from build123d import *

# Parameters (mm, degrees)
SKETCH1_R           = 43.2435
BOSS_EXTRUDE1_DEPTH = 1.5875


with BuildPart() as part:
    # Sketch1 → Boss-Extrude1 (new body)
    with BuildSketch(Plane.XY):
        Circle(SKETCH1_R)
        with BuildLine():
            Line((39.84498, 0.79375), (39.84498, -0.79375))
            Line((39.84498, -0.79375), (31.740076574, -0.79375))
            ThreePointArc((31.740076574, -0.79375), (0, -31.75), (-31.740076574, -0.79375))
            Line((-31.740076574, -0.79375), (-39.84498, -0.79375))
            Line((-39.84498, -0.79375), (-39.84498, 0.79375))
            Line((-39.84498, 0.79375), (-31.740076574, 0.79375))
            ThreePointArc((-31.740076574, 0.79375), (0, 31.75), (31.740076574, 0.79375))
            Line((31.740076574, 0.79375), (39.84498, 0.79375))
        make_face(mode=Mode.SUBTRACT)
    extrude(amount=BOSS_EXTRUDE1_DEPTH)


solid = part.part
Input: part model. Units: mm. Frame: model coordinates. A direction names the side the tool comes from. Give positions to 0.01 mm unless a question says otherwise; leave off trailing zeros. Order: outer loops, then holes, each group sorted by start corner. A loop starts at its lowest first (then second) coordinate and runs counter-clockwise, first axis right, second up. Notation, with made-up numbers: (20.5, -11.75) - (64.5, -11.75) arc R15 cw to (64.5, 5.25) - close; hole circle Ø1 at (-7.5, -25). An arc over 180 degrees is marked (long way). Answer as a JSON object with one key per item and string values. Group by question number.
Q1. Cut plane B-B, the plane x = 0. Output: boundary loops of the cut face in (y, z), then the cut area to 3 significant figures.
Q2. Cut plane C-C, the plane y = 5. Output: boundary loops of the cut face in (x, z).
Q3. Line query: probe 1 along Y at (x, z) = (34, 1.25); probe 2 along X at (y, z) = (-14, 0.3); probe 3 along X at (y, z) = (17, 0.7). Output: solid intervals per line, ascending.
Q4. Set-up query: faces 1 (the face through (-0.687, 31.743, 0.783)), 2 (the face through (0, 32, 0)). Return all of +Z, -Z, +X, -X, +Y, -Y with unobstructed straight access to the full face (end or side cutting, diameter ignored); none if empty.
Q5. Mould query, pull axis Y, two halves, no side actions, for faces 3 (the face through (0, 32, 1.588)), 4 (the face through (23.25, 36.46, 0.78)), 5 (the face through (0.687, -31.743, 0.783)). Classes: pulls with the +Y half, pulls with the -Y half, needs draft (parallel to the pull), parting line crosses it, or undercut.
Q6. Cut plane A-A, the plane z = 1.2. Output: boundary loops of the cut face in (x, y), then the cut area to 3 significant figures.
Q7. First-contact query: pin 1 Ø0.8 at (x, z) = (37, 1) entering from +Y. Flat tip, straight axial feed; report the tip coordinate or a pass-through.
Results:
{
 "1": {"outline": "(-43.24, 0) - (-31.75, 0) - (-31.75, 1.59) - (-43.24, 1.59) - close; (31.75, 0) - (43.24, 0) - (43.24, 1.59) - (31.75, 1.59) - close", "area": "36.5 mm^2"},
 "2": {"outline": "(-42.95, 0) - (-31.35, 0) - (-31.35, 1.59) - (-42.95, 1.59) - close; (31.35, 0) - (42.95, 0) - (42.95, 1.59) - (31.35, 1.59) - close"},
 "3": {"probe 1": "-26.72 to -0.79, 0.79 to 26.72", "probe 2": "-40.91 to -28.5, 28.5 to 40.91", "probe 3": "-39.76 to -26.82, 26.82 to 39.76"},
 "4": {"face 1": "+Z, -Z", "face 2": "-Z, +X, -X, +Y, -Y"},
 "5": {"face 3": "needs draft", "face 4": "parting line crosses it", "face 5": "undercut"},
 "6": {"outline": "circle Ø86.49 at (0, 0); hole (-39.84, -0.79) - (-31.74, -0.79) arc R31.75 ccw to (31.74, -0.79) - (39.84, -0.79) - (39.84, 0.79) - (31.74, 0.79) arc R31.75 ccw to (-31.74, 0.79) - (-39.84, 0.79) - close", "area": "2,680 mm^2"},
 "7": {"pin 1": "y = 23.03"}
}
